from build123d import *

# Parameters (mm, degrees)
SKETCH1_R           = 2.4
SKETCH1_R_2         = 2
BOSS_EXTRUDE1_DEPTH = 2
BOSS_EXTRUDE2_START = 2
SKETCH1_3_R         = 2.4
BOSS_EXTRUDE2_DEPTH = 12


with BuildPart() as part:
    # Sketch1 → Boss-Extrude1 (new body)
    # profile 1 of 4: a face of its own
    with BuildSketch(Plane(origin=(0, 0, 0), x_dir=(1, 0, 0), z_dir=(0, 1, 0))):
        with BuildLine():
            ThreePointArc((22.083647797, -7.75), (4.330127019, 2.5), (4.330127019, 23))
            ThreePointArc((4.330127019, 23), (4.760296424, 23.970432103), (4.975912761, 25.009803922))
            ThreePointArc((4.975912761, 25.009803922), (0, 30.5), (-4.975912761, 25.009803922))
            ThreePointArc((-4.975912761, 25.009803922), (-4.760296424, 23.970432103), (-4.330127019, 23))
            ThreePointArc((-4.330127019, 23), (-2.282168358, 18.055790425), (-1.583647797, 12.75))
            ThreePointArc((-1.583647797, 12.75), (-7.587958782, -1.745689014), (-22.083647797, -7.75))
            ThreePointArc((-22.083647797, -7.75), (-23.139151353, -7.862678418), (-24.14708192, -8.195635103))
            ThreePointArc((-24.14708192, -8.195635103), (-26.413774815, -15.25), (-19.171169159, -16.814168819))
            ThreePointArc((-19.171169159, -16.814168819), (-18.378854928, -16.107753684), (-17.753520778, -15.25))
            ThreePointArc((-17.753520778, -15.25), (0, -5), (17.753520778, -15.25))
            ThreePointArc((17.753520778, -15.25), (18.378854928, -16.107753684), (19.171169159, -16.814168819))
            ThreePointArc((19.171169159, -16.814168819), (26.413774815, -15.25), (24.14708192, -8.195635103))
            ThreePointArc((24.14708192, -8.195635103), (23.139151353, -7.862678418), (22.083647797, -7.75))
        make_face()
        with Locations((-22.083647797, -12.75)):
            Circle(SKETCH1_R, mode=Mode.SUBTRACT)
        with Locations((22.083647797, -12.75)):
            Circle(SKETCH1_R, mode=Mode.SUBTRACT)
        with Locations(Location((0, 0, 0), (0, 0, 270))):
            Circle(SKETCH1_R_2, mode=Mode.SUBTRACT)
        with Locations((0, 25.5)):
            Circle(SKETCH1_R, mode=Mode.SUBTRACT)
    # profile 2 of 4: a face of its own
    with BuildSketch(Plane(origin=(0, 0, 0), x_dir=(1, 0, 0), z_dir=(0, 1, 0))):
        with Locations((-22.083647797, -12.75)):
            Circle(SKETCH1_R)
    # profile 3 of 4: a face of its own
    with BuildSketch(Plane(origin=(0, 0, 0), x_dir=(1, 0, 0), z_dir=(0, 1, 0))):
        with Locations((22.083647797, -12.75)):
            Circle(SKETCH1_R)
    # profile 4 of 4: a face of its own
    with BuildSketch(Plane(origin=(0, 0, 0), x_dir=(1, 0, 0), z_dir=(0, 1, 0))):
        with Locations((0, 25.5)):
            Circle(SKETCH1_R)
    extrude(amount=BOSS_EXTRUDE1_DEPTH)

    # Sketch1<3> → Boss-Extrude2 (add)
    with BuildSketch(Plane(origin=(0, 0, 0), x_dir=(1, 0, 0), z_dir=(0, 1, 0)).offset(BOSS_EXTRUDE2_START)):
        with Locations(Location((-22.083647797, -12.75, 0), (0, 0, 270))):
            Circle(SKETCH1_3_R)
        with Locations(Location((22.083647797, -12.75, 0), (0, 0, 270))):
            Circle(SKETCH1_3_R)
        with Locations(Location((0, 25.5, 0), (0, 0, 270))):
            Circle(SKETCH1_3_R)
    extrude(amount=BOSS_EXTRUDE2_DEPTH)


solid = part.part
Part model, mm, in its own coordinate system. A direction names the side the tool comes from. Coordinates: 2 decimals unless noted, no trailing zeros. Order: outer loops, then holes, each group sorted by start corner. A loop starts at its lowest first (then second) coordinate and runs counter-clockwise, first axis right, second up. Notation, with made-up numbers: M 55,56 L 105,56 A20 ccw 105,94 Z; hole C 77.25,-10 d10. An arc over 180 degrees is marked long. One line per question, with ' | ' between items.
Q1. Pin check, flat tips, straight feed: P1, Ø3.5, axis at x = 0, z = 0, coming from the +Y side; P2, Ø8, axis at x = -20.5, y = 4, coming from the -Z side; P3, Ø14.5, axis at x = 7, z = 1.5, coming from the +Y side. Stop position of each tip, or through.
A:
P1: passes through | P2: stops at z = 7.12 | P3: stops at y = 2
Q2. Drill centre lines: line 1 (Y direction, x = 14, z = 7); line 2 (X direction, y = 0.45, z = 0); line 3 (X direction, y = 10.75, z = 11). Where is each one in solid material? Low to high.
A:
line 1: y = 0 to 2 | line 2: x = -6.03 to -2, 2 to 6.03 | line 3: x = -23.73 to -20.44, 20.44 to 23.73
Q3. Slice it at B-B (z = 0). Give the cut face in (x, y).
A:
outline: M -6.03,0 L -2,0 L -2,2 L -6.03,2 Z; M 2,0 L 6.03,0 L 6.03,2 L 2,2 Z
Q4. Two-plate mould, pull along Z, no slides. Class faces 1 (the face through (2, 0, -1)), 2 (the face through (-2, 1, 0)), 3 (the face through (0, 1, 5)), 4 (the face through (0.106, 7.916, -27.898)): +Z half, -Z half, draft (parallel to the pull), parting line (faces both ways), or undercut.
A:
face 1: draft | face 2: undercut | face 3: +Z half | face 4: parting line
Q5. 3-axis set-ups, long thin cutter, end or side, ignore diameter. For faces 5 (the face through (22, 14, 13)), 6 (the face through (24.463, 7.916, 12.438)): which of +Z, -Z, +X, -X, +Y, -Y reach the whole face in a straight line?
A:
face 5: +Z, -Z, +X, -X, +Y | face 6: +Y
Q6. Slice it at D-D (z = 12.75). Give the cut face in (x, y).
A:
outline: M -27.08,0 L -16.05,0 L -16.05,2 L -19.68,2 L -19.68,14 L -24.48,14 L -24.48,2 L -27.08,2 Z; M 16.05,0 L 27.08,0 L 27.08,2 L 24.48,2 L 24.48,14 L 19.68,14 L 19.68,2 L 16.05,2 Z
Q7. Slice it at A-A (x = 0). Give the cut face in (y, z), and give its area (3 significant figures).
A:
outline: M 0,-30.5 L 2,-30.5 L 2,-27.9 L 14,-27.9 L 14,-23.1 L 2,-23.1 L 2,-2 L 0,-2 Z; M 0,2 L 2,2 L 2,5 L 0,5 Z | area: 121 mm^2
Q8. Slice it at C-C (y = 3.5). Give the cut face in (x, z).
A:
outline: C -22.08,12.75 d4.8; C 0,-25.5 d4.8; C 22.08,12.75 d4.8
